```python
from build123d import *

# Parameters (mm, degrees)
SKETCH1_R          = 2.4
EXTRUDE_269_DEPTH  = 3.5
EXTRUDE_450_DEPTH  = 4.5
SKETCH3_W          = 22.5
SKETCH3_H          = 12
EXTRUDE_686_DEPTH  = 23.2
SKETCH4_W          = 32.2
SKETCH4_H          = 12
EXTRUDE_857_DEPTH  = 2.5
SKETCH5_R          = 1.25
CUT_EXTRUDE1_DEPTH = 36.483975256


with BuildPart() as part:
    # Sketch1 → Extrude 269 (new body)
    with BuildSketch(Plane(origin=(0, 0, 0), x_dir=(1, 0, 0), z_dir=(0, 1, 0))):
        with Locations(Location((0, 0, 0), (0, 0, 270))):
            Circle(SKETCH1_R)
    extrude(amount=EXTRUDE_269_DEPTH)

    # Sketch2 → Extrude 450 (add)
    with BuildSketch(Plane(origin=(0, 0, 0), x_dir=(1, 0, 0), z_dir=(0, 1, 0))):
        with BuildLine():
            Line((5.85, -2.85), (5.279914772, -2.85))
            ThreePointArc((5.279914772, -2.85), (-6, 0), (5.279914772, 2.85))
            Line((5.279914772, 2.85), (5.85, 2.85))
            ThreePointArc((5.85, 2.85), (8.7, 0), (5.85, -2.85))
        make_face()
    extrude(amount=-EXTRUDE_450_DEPTH)

    # Sketch3 → Extrude 686 (add)
    with BuildSketch(Plane(origin=(0, -4.5, 0), x_dir=(-1, 0, 0), z_dir=(0, -1, 0))):
        with Locations((-5.25, 0)):
            Rectangle(SKETCH3_W, SKETCH3_H)
    extrude(amount=EXTRUDE_686_DEPTH)

    # Sketch4 → Extrude 857 (add)
    with BuildSketch(Plane(origin=(0, -8.5, 0), x_dir=(1, 0, 0), z_dir=(0, 1, 0))):
        with Locations((5.25, 0)):
            Rectangle(SKETCH4_W, SKETCH4_H)
    extrude(amount=-EXTRUDE_857_DEPTH)

    # Sketch5 → Cut-Extrude1 (cut, through all)
    with BuildSketch(Plane(origin=(0, 0, 0), x_dir=(1, 0, 0), z_dir=(0, 1, 0))):
        with Locations(Location((-8.55, 0, 0), (0, 0, 90))):
            Circle(SKETCH5_R)
        with Locations(Location((19.05, 0, 0), (0, 0, 90))):
            Circle(SKETCH5_R)
    extrude(amount=-CUT_EXTRUDE1_DEPTH, mode=Mode.SUBTRACT)


solid = part.part
```
Work out the finished part from the listing and answer in its coordinate system (mm). A direction names the side the tool comes from. Round coordinates to 2 decimals unless told otherwise and drop trailing zeros. Write each loop counter-clockwise with the first axis right and the second up, starting at its lowest first coordinate (ties: lowest second). Pieces come first, ordered by that corner, then holes. Notation, with made-up numbers: (54, -27.5) -> (61, -27.5) arc R26 cw to (61, 11.5) -> close; hole circle Ø3 at (12.5, 10.5). An arc over 180 degrees is marked (long way). Write each question's results on one line, items separated by ' | '.
1) The part is cut by section A-A (x = -8.55). Write down the section's boundary in (y, z), and give its area (4 significant figures).
Findings:
outline: (-11, -6) -> (-8.5, -6) -> (-8.5, -1.25) -> (-11, -1.25) -> close; (-11, 1.25) -> (-8.5, 1.25) -> (-8.5, 6) -> (-11, 6) -> close | area: 23.75 mm²
2) Which of the six approach directions +Z, -Z, +X, -X, +Y, -Y give full straight-line access (tool end or side, diameter ignored) to faces 1 (the flat face through (-5, -4.5, -5)), 2 (the flat face through (-8.5, -11, -1.4)), 3 (the flat face through (16.5, -6, 0)), 4 (the flat face through (10, -4.5, 0))?
Findings:
face 1: -Z, -X, +Y | face 2: +Z, -Z, -X, -Y | face 3: +Z, -Z, +X, +Y | face 4: +X, +Y
3) Consider line 1 along X through (y, z) = (-9.7, 0); line 2 along Z through (x, y) = (19.05, -10.05); line 3 along X through (y, z) = (-8, -3). Determine where each line is inside the solid, lowest interval first. Write a range as [from, to].
Findings:
line 1: x = [-10.85, -9.8], [-7.3, 17.8], [20.3, 21.35] | line 2: z = [-6, -1.25], [1.25, 6] | line 3: x = [-6, 16.5]
4) Flat-ended cylindrical pins translate along their axes: pin 1 (2.5 mm diameter, centred on x = 18, z = 0, fed in from +Y); pin 2 (6 mm diameter, centred on y = -21.5, z = -2.5, fed in from +X); pin 3 (2 mm diameter, centred on y = -5.5, z = 1, fed in from -X). Find the tip coordinate at first contact, or state that the pin passes through.
Findings:
pin 1: stops at y = -8.5 | pin 2: stops at x = 16.5 | pin 3: stops at x = -6
5) The part is cut by section B-B (y = -9.5). Write down the section's boundary in (x, z).
Findings:
outline: (-10.85, -6) -> (21.35, -6) -> (21.35, 6) -> (-10.85, 6) -> close; hole circle Ø2.5 at (-8.55, 0); hole circle Ø2.5 at (19.05, 0)
6) The part is cut by section C-C (z = -1.75). Write down the section's boundary in (x, y).
Findings:
outline: (-10.85, -11) -> (-6, -11) -> (-6, -27.7) -> (16.5, -27.7) -> (16.5, -11) -> (21.35, -11) -> (21.35, -8.5) -> (16.5, -8.5) -> (16.5, -4.5) -> (8.1, -4.5) -> (8.1, 0) -> (1.64, 0) -> (1.64, 3.5) -> (-1.64, 3.5) -> (-1.64, 0) -> (-5.74, 0) -> (-5.74, -4.5) -> (-6, -4.5) -> (-6, -8.5) -> (-10.85, -8.5) -> close
7) The part is cut by section D-D (x = -3). Write down the section's boundary in (y, z), and give its area (3 significant figures).
Findings:
outline: (-27.7, -6) -> (-4.5, -6) -> (-4.5, -5.2) -> (0, -5.2) -> (0, 5.2) -> (-4.5, 5.2) -> (-4.5, 6) -> (-27.7, 6) -> close | area: 325 mm²
8) For a pull along Z with two mould halves and no side action, classify faces 5 (the cylindrical face through (17.996, -9.732, -0.672)), 6 (the flat face through (5, -16, 6)), 7 (the flat face through (16.5, -19, 0)) as +Z half, -Z half, draft (parallel to the pull), parting line (faces both ways), or undercut.
Findings:
face 5: undercut | face 6: +Z half | face 7: draft
